```python
from build123d import *

# Parameters (mm, degrees)
SKETCH1_W           = 93
SKETCH1_H           = 90
BOSS_EXTRUDE2_DEPTH = 120
SKETCH4_W           = 83.188465172
SKETCH4_H           = 100
CUT_EXTRUDE2_DEPTH  = 86
SKETCH6_W           = 85.554409806
SKETCH6_H           = 11
CUT_EXTRUDE4_DEPTH  = 86
CUT_EXTRUDE5_START  = -10
SKETCH8_W           = 74.401519334
SKETCH8_H           = 6.478481014
CUT_EXTRUDE5_DEPTH  = 50


with BuildPart() as part:
    # Sketch1 → Boss-Extrude2 (new body)
    with BuildSketch(Plane(origin=(0, 0, 0), x_dir=(1, 0, 0), z_dir=(0, 1, 0))):
        Rectangle(SKETCH1_W, SKETCH1_H)
    extrude(amount=BOSS_EXTRUDE2_DEPTH)

    # Sketch4 → Cut-Extrude2 (cut)
    with BuildSketch(Plane.XY.offset(45)):
        with Locations((-4.905767414, 52.095291963)):
            Rectangle(SKETCH4_W, SKETCH4_H)
    extrude(amount=-CUT_EXTRUDE2_DEPTH, mode=Mode.SUBTRACT)

    # Sketch6 → Cut-Extrude4 (cut)
    with BuildSketch(Plane(origin=(46.5, 0, 0), x_dir=(0, 0, -1), z_dir=(1, 0, 0))):
        with Locations((0.366871397, 111.285550359)):
            Rectangle(SKETCH6_W, SKETCH6_H)
    extrude(amount=-CUT_EXTRUDE4_DEPTH, mode=Mode.SUBTRACT)

    # Sketch8 → Cut-Extrude5 (cut)
    with BuildSketch(Plane.ZY.offset(46.5).offset(CUT_EXTRUDE5_START)):
        with Locations((1.540859868, 105.33453247)):
            Rectangle(SKETCH8_W, SKETCH8_H)
    extrude(amount=-CUT_EXTRUDE5_DEPTH, mode=Mode.SUBTRACT)


solid = part.part
```
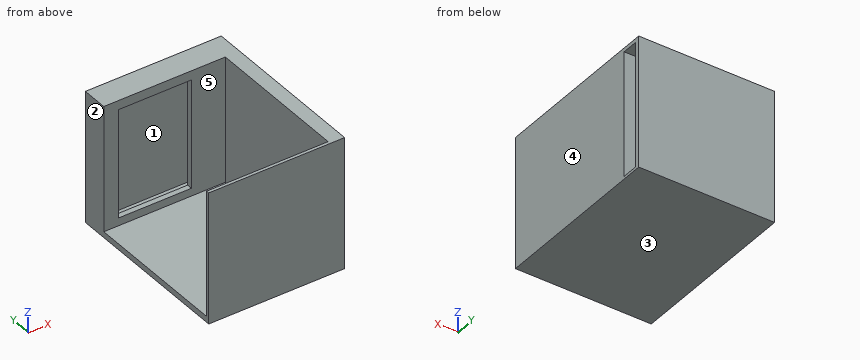
The listing builds one solid part. Answer for the finished solid, in the listing's coordinates (mm). Face numbers are marked on the shaded views. A direction names the side the tool comes from. Round coordinates to 2 decimals unless told otherwise and drop trailing zeros. Loops run counter-clockwise (first coordinate to the right, second up) from the corner with the lowest first, then second, coordinate; pieces in that order, holes last. Notation, with made-up numbers: (73, 0.25) - (122, 0.25) arc R33 ccw to (122, 33.25) - close; hole circle Ø4 at (-6, 79.25). An arc over 180 degrees is marked (long way). Use one line per item in the form item = value. Start each with the question number.
1. Given pin 1 Ø6 at (x, z) = (-24, 1) entering from -Y, flat-ended and moving along its own axis, determine where the tip first touches the part or whether it passes through.
2. The part is cut by section C-C on x = -9.5. Determine the outline of the cut face in (y, z), then the cut area to 3 significant figures.
3. A tool of negligible diameter and unlimited length cuts with its end or side. For the marked faces 4 and 5, from which of +Z, -Z, +X, -X, +Y, -Y can it reach the whole face along a straight path? Write none if from no direction.
4. The part is cut by section D-D on y = 65. Determine the outline of the cut face in (x, z).
5. For a pull along Z with two mould halves and no side action, classify the marked faces 1, 2 and 3 as pulls with the +Z half, pulls with the -Z half, needs draft (parallel to the pull), parting line crosses it, or undercut.
6. The part is cut by section A-A on z = -13.5. Determine the outline of the cut face in (x, y), then the cut area to 3 significant figures.
7. The part is cut by section B-B on x = 33. Determine the outline of the cut face in (y, z), then the cut area to 3 significant figures.
8. Consider line 1 (Y direction, x = 20, z = 4); line 2 (Y direction, x = 37, z = -26); line 3 (Y direction, x = -2.5, z = 10.5). Determine where each line is inside the solid, lowest interval first. Write a range as [from, to].
Geometry check:
q1.pin_1 = 0
q2.outline = (0, -45) - (120, -45) - (120, 45) - (102.1, 45) - (102.1, 38.74) - (105.79, 38.74) - (105.79, 42.41) - (116.79, 42.41) - (116.79, -43.14) - (105.79, -43.14) - (105.79, -35.66) - (102.1, -35.66) - (102.1, -41) - (2.1, -41) - (2.1, 45) - (0, 45) - close
q2.area = 984 mm^2
q3.face_4 = +Z, -Z, +X, +Y, -Y
q3.face_5 = +Z, -X
q4.outline = (-46.5, -45) - (46.5, -45) - (46.5, 45) - (36.69, 45) - (36.69, -41) - (-46.5, -41) - close
q5.face_1 = undercut
q5.face_2 = needs draft
q5.face_3 = pulls with the -Z half
q6.outline = (-46.5, 0) - (46.5, 0) - (46.5, 105.79) - (13.5, 105.79) - (13.5, 102.1) - (36.69, 102.1) - (36.69, 2.1) - (-46.5, 2.1) - close; (-46.5, 102.1) - (-36.5, 102.1) - (-36.5, 105.79) - (-39.5, 105.79) - (-39.5, 116.79) - (46.5, 116.79) - (46.5, 120) - (-46.5, 120) - close
q6.area = 1,710 mm^2
q7.outline = (0, -45) - (120, -45) - (120, 45) - (102.1, 45) - (102.1, -41) - (2.1, -41) - (2.1, 45) - (0, 45) - close; hole (105.79, -43.14) - (116.79, -43.14) - (116.79, 42.41) - (105.79, 42.41) - close
q7.area = 1,260 mm^2
q8.line_1 = [0, 2.1], [102.1, 105.79], [116.79, 120]
q8.line_2 = [0, 105.79], [116.79, 120]
q8.line_3 = [0, 2.1], [116.79, 120]
